from build123d import *

# Parameters (mm, degrees)
F0_W     = 94.1855311394
F0_H     = 52.4866655469
F1_DEPTH = 90
F4_D     = 20
F4_DEPTH = 80
F4_TIP   = 6.0086061903
F5_R     = 9.112196694
F7_DEPTH = 80


# Not quite as in the source:
# - the program builds the solid bodies; features that only make, move or delete a surface that nothing else refers to are left out


with BuildPart() as f1:
    # F0 (on Front) → F1 (new body)
    with BuildSketch(Plane.XZ):
        with Locations((9.957909584, -2.3857913911)):
            Rectangle(F0_W, F0_H)
    extrude(amount=F1_DEPTH)

    # F4
    with Locations(Plane.XZ.offset(90)):
        with Locations((28.2388776541, 0)):
            Hole(F4_D / 2, depth=F4_DEPTH)
            with Locations((0, 0, -(F4_DEPTH + F4_TIP / 2))):  # 118° drill point
                Cone(0, F4_D / 2, F4_TIP, mode=Mode.SUBTRACT)

    # F5 (on face) → F7 (cut)
    with BuildSketch(Plane.XZ.offset(90)):
        with Locations((-17.2343160957, 0)):
            Circle(F5_R)
    extrude(amount=F7_DEPTH, mode=Mode.SUBTRACT)


solid = f1.part
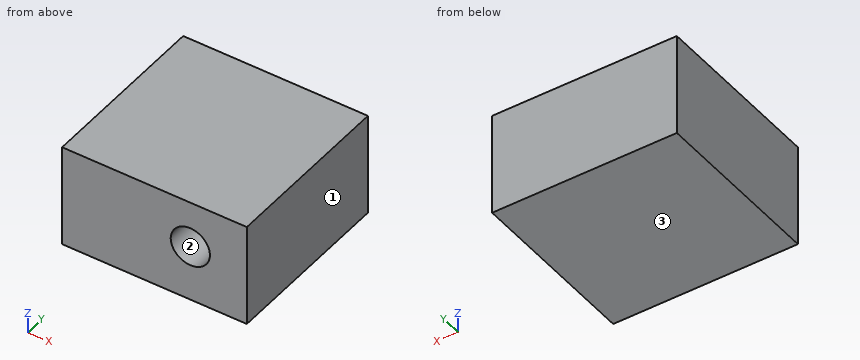
Verification items for the finished model (mm, model axes). Face numbers are marked on the shaded views. Round coordinates to 2 decimals unless told otherwise and drop trailing zeros. Write each loop counter-clockwise with the first axis right and the second up, starting at its lowest first coordinate (ties: lowest second). Pieces come first, ordered by that corner, then holes.
(1) Mould release check, pull along X, two halves, no side actions. Record for the marked faces 1, 2 and 3: pulls with the +X half, pulls with the -X half, needs draft (parallel to the pull), parting line crosses it, or undercut.
Returned:
face 1: pulls with the +X half
face 2: undercut
face 3: needs draft
(2) Section check A-A (y = -15). Enter the section's corners in (x, z), plus the area to 3 significant figures.
Returned:
outline: (-37.13, -28.63) - (57.05, -28.63) - (57.05, 23.86) - (-37.13, 23.86) - close; hole circle Ø20 at (28.24, 0)
area: 4,630 mm2
(3) Material ranges on line 1 (X direction, y = -68.5, z = 0); line 2 (X direction, y = -53.5, z = 3); line 3 (Z direction, x = 25, y = -33.5), recorded low to high.
Returned:
line 1: x = -37.13 to 18.24, 38.24 to 57.05
line 2: x = -37.13 to 18.7, 37.78 to 57.05
line 3: z = -28.63 to -9.46, 9.46 to 23.86
